Build history of the part. All positions in model axes, mm. Coordinates: 2 decimals unless noted, no trailing zeros. Loops run counter-clockwise (first coordinate to the right, second up) from the corner with the lowest first, then second, coordinate; pieces in that order, holes last.
Item 1: Cut at D-D (x = 0). List the corners of the cut face in (y, z), and give its area (3 significant figures).
Item 2: Cut at A-A (y = 0). List the corners of the cut face in (x, z), and give its area (3 significant figures).
Item 3: Drill centre lines: line 1 along Y through (x, z) = (120, -1.3); line 2 along X through (y, z) = (0.25, -3.15); line 3 along Y through (x, z) = (46, -3.75). Where is each one in solid material? Low to high.
Item 4: Cut at B-B (x = 120). List the corners of the cut face in (y, z), and give its area (3 significant figures).
Item 5: Flat gauge pins, fed straight in: pin 1 (2.5 mm diameter, centred on x = 44.5, z = -2.5, fed in from -Y); pin 2 (1.5 mm diameter, centred on y = -5.5, z = -3.5, fed in from +X). Where does each tip first touch, or does it go through?
Item 6: Cut at C-C (z = -1.55). List the corners of the cut face in (x, y), and give its area (3 significant figures).
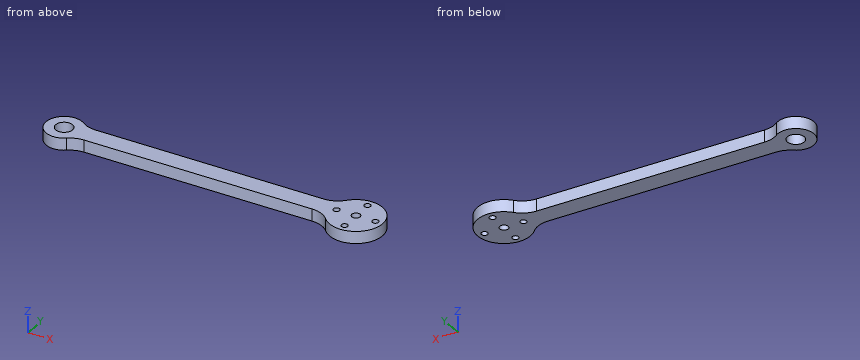
from build123d import *

# Parameters (mm, degrees)
SKETCH1_R          = 3.5
SKETCH1_R_2        = 1.3
SKETCH1_R_3        = 1.75
BASE_FLANGE1_DEPTH = 5
FILLET1_R          = 10
FILLET2_R          = 10


# Sheet-metal steps are written as plain solids
with BuildPart() as part:
    # Sketch1 → Base-Flange1 (new body)
    with BuildSketch(Plane.XY):
        with BuildLine():
            Line((6.34428877, 4), (109.753049234, 4))
            ThreePointArc((109.753049234, 4), (131, 0), (109.753049234, -4))
            Line((109.753049234, -4), (6.34428877, -4))
            ThreePointArc((6.34428877, -4), (-7.5, 0), (6.34428877, 4))
        make_face()
        Circle(SKETCH1_R, mode=Mode.SUBTRACT)
        with Locations((112, 0)):
            Circle(SKETCH1_R_2, mode=Mode.SUBTRACT)
        with Locations((120, -8)):
            Circle(SKETCH1_R_2, mode=Mode.SUBTRACT)
        with Locations((128, 0)):
            Circle(SKETCH1_R_2, mode=Mode.SUBTRACT)
        with Locations((120, 8)):
            Circle(SKETCH1_R_2, mode=Mode.SUBTRACT)
        with Locations((120, 0)):
            Circle(SKETCH1_R_3, mode=Mode.SUBTRACT)
    extrude(amount=-BASE_FLANGE1_DEPTH)

    # Fillet1
    fillet1_edges = [part.edges().sort_by_distance(p)[0] for p in [
        (6.34428877, 4, -2.5),
        (6.34428877, -4, -2.5),
    ]]
    fillet(fillet1_edges, radius=FILLET1_R)

    # Fillet2
    fillet2_edges = [part.edges().sort_by_distance(p)[0] for p in [
        (109.753049234, 4, -2.5),
        (109.753049234, -4, -2.5),
    ]]
    fillet(fillet2_edges, radius=FILLET2_R)


solid = part.part
Filled sheet:
1. outline: (-7.5, -5) - (-3.5, -5) - (-3.5, 0) - (-7.5, 0) - close; (3.5, -5) - (7.5, -5) - (7.5, 0) - (3.5, 0) - close
1. area: 40.0 mm2
2. outline: (-7.5, -5) - (-3.5, -5) - (-3.5, 0) - (-7.5, 0) - close; (3.5, -5) - (110.7, -5) - (110.7, 0) - (3.5, 0) - close; (113.3, -5) - (118.25, -5) - (118.25, 0) - (113.3, 0) - close; (121.75, -5) - (126.7, -5) - (126.7, 0) - (121.75, 0) - close; (129.3, -5) - (131, -5) - (131, 0) - (129.3, 0) - close
2. area: 614 mm2
3. line 1: y = -11 to -9.3, -6.7 to -1.75, 1.75 to 6.7, 9.3 to 11
3. line 2: x = -7.5 to -3.49, 3.49 to 110.72, 113.28 to 118.27, 121.73 to 126.72, 129.28 to 131
3. line 3: y = -4 to 4
4. outline: (-11, -5) - (-9.3, -5) - (-9.3, 0) - (-11, 0) - close; (-6.7, -5) - (-1.75, -5) - (-1.75, 0) - (-6.7, 0) - close; (1.75, -5) - (6.7, -5) - (6.7, 0) - (1.75, 0) - close; (9.3, -5) - (11, -5) - (11, 0) - (9.3, 0) - close
4. area: 66.5 mm2
5. pin 1: stops at y = -4
5. pin 2: stops at x = 129.92
6. outline: (4.5, -6) arc R10 cw to (10.5, -4) - (104.35, -4) arc R10 cw to (111.8, -7.33) arc R11 ccw (long way) to (111.8, 7.33) arc R10 cw to (104.35, 4) - (10.5, 4) arc R10 cw to (4.5, 6) arc R7.5 ccw (long way) to start; hole circle Ø7 at (0, 0); hole circle Ø2.6 at (112, 0); hole circle Ø3.5 at (120, 0); hole circle Ø2.6 at (120, -8); hole circle Ø2.6 at (120, 8); hole circle Ø2.6 at (128, 0)
6. area: 1,320 mm2
